from build123d import *

# Parameters (mm, degrees)
F1_DEPTH = 63.5
F0_W     = 25.4
F0_H     = 19.05
F0_H_2   = 9.525
F2_DEPTH = 25.4
F3_DEPTH = 7.9375
F5_R     = 6.35


with BuildPart() as f1:
    # F0 (on Front) → F1 (new body, symmetric)
    with BuildSketch(Plane.XZ):
        Polygon((-41.275, -9.525), (41.275, -9.525), (41.275, 9.525), (22.2237235206, 9.525), (-41.275, 9.525), align=None)
    extrude(amount=F1_DEPTH, both=True)

    # F0 (on Front) → F2 (join, symmetric)
    with BuildSketch(Plane.XZ):
        with BuildLine():
            Line((22.2237235206, 9.525), (41.275, 9.525))
            Line((41.275, 9.525), (40.9650549741, 36.2983668991))
            ThreePointArc((40.9650549741, 36.2983668991), (47.6329246689, 41.7219107909), (56.1502739404, 42.8752))
            Line((56.1502739404, 42.8752), (60.325, 42.8752))
            Line((60.325, 42.8752), (60.325, 61.9252))
            Line((60.325, 61.9252), (50.6626719245, 61.9252))
            ThreePointArc((50.6626719245, 61.9252), (33.3863605767, 55.3894970066), (21.8598589674, 40.95599057))
            Line((21.8598589674, 40.95599057), (22.2237235206, 9.525))
        make_face()
        with Locations((73.025, 52.4002)):
            Rectangle(F0_W, F0_H)
        with Locations((73.025, 38.1127)):
            Rectangle(F0_W, F0_H_2)
    extrude(amount=F2_DEPTH, both=True)

    # F0 (on Front) → F3 (join, symmetric)
    with BuildSketch(Plane.XZ):
        with BuildLine():
            add(Edge.make_bspline(
                [(-41.275, 9.525), (-56.7215932498, 57.9155711565), (13.6268828042, 66.4033379321), (50.6626719245, 61.9252)],
                knots=[0, 0, 0, 0, 105.8220982543, 105.8220982543, 105.8220982543, 105.8220982543], degree=3))
            Line((-41.275, 9.525), (22.2237235206, 9.525))
            Line((22.2237235206, 9.525), (21.8598589674, 40.95599057))
            ThreePointArc((21.8598589674, 40.95599057), (33.3863605767, 55.3894970066), (50.6626719245, 61.9252))
        make_face()
    extrude(amount=F3_DEPTH, both=True)

    # F0 (on Front) → F4 (revolve)
    with BuildSketch(Plane.XZ):
        Polygon((111.125, 61.9252), (85.725, 61.9252), (85.725, 42.8752), (85.725, 33.3502), (111.125, 33.3502), align=None)
    revolve(axis=Axis((85.725, 0, 52.4002), (0, 0, -1)))

    # F5
    f5_edges = [f1.edges().sort_by_distance(p)[0] for p in [
        (41.275, 63.5, 0),
        (-41.275, 63.5, 0),
        (-41.275, -63.5, 0),
        (41.275, -63.5, 0),
    ]]
    fillet(f5_edges, radius=F5_R)


solid = f1.part
Input: part model. Units: mm. Frame: model coordinates. A direction names the side the tool comes from. Round coordinates to 2 decimals unless told otherwise and drop trailing zeros. Order: outer loops, then holes, each group sorted by start corner. A loop starts at its lowest first (then second) coordinate and runs counter-clockwise, first axis right, second up. Notation, with made-up numbers: (29, -10.5) - (77, -10.5) arc R21 cw to (77, 25.5) - close; hole circle Ø6 at (50, 29.5). An arc over 180 degrees is marked (long way). Use a Markdown table: item, result.
1. Section A-A on y = 12. Return the cut outline in (x, z) (3 decimals).
Evaluation:
| item | result |
|---|---|
| outline | (-41.275, -9.525) - (41.275, -9.525) - (41.275, 9.525) - (40.965, 36.298) arc R15.875 cw to (56.15, 42.875) - (60.325, 42.875) - (60.325, 33.35) - (108.112, 33.35) - (108.112, 61.925) - (50.663, 61.925) arc R34.925 ccw to (21.86, 40.956) - (22.224, 9.525) - (-41.275, 9.525) - close |
2. First-contact query: pin 1 (1 mm diameter, centred on x = 52.5, z = 41, fed in from -Y); pin 2 (8 mm diameter, centred on x = 43.5, y = -4, fed in from +Z); pin 3 (1.5 mm diameter, centred on y = 25, z = 32.5, fed in from -X); pin 4 (21 mm diameter, centred on y = 25.5, z = 0, fed in from -X) (3 decimals). Flat tips, straight axial feed; report the tip coordinate or a pass-through.
Evaluation:
| item | result |
|---|---|
| pin 1 | through |
| pin 2 | z = 62.82 |
| pin 3 | x = 21.95 |
| pin 4 | x = -41.275 |
3. Section C-C on x = 63.5. Return the cut outline in (y, z), then the cut area to 3 significant figures.
Evaluation:
| item | result |
|---|---|
| outline | (-25.4, 33.35) - (25.4, 33.35) - (25.4, 61.93) - (-25.4, 61.93) - close |
| area | 1,450 mm^2 |
4. Section D-D on y = -38. Return the cut outline in (x, z) (3 decimals).
Evaluation:
| item | result |
|---|---|
| outline | (-41.275, -9.525) - (41.275, -9.525) - (41.275, 9.525) - (-41.275, 9.525) - close |
5. Section B-B on z = -3.5. Return the cut outline in (x, y) (3 decimals).
Evaluation:
| item | result |
|---|---|
| outline | (-41.275, -57.15) arc R6.35 ccw to (-34.925, -63.5) - (34.925, -63.5) arc R6.35 ccw to (41.275, -57.15) - (41.275, 57.15) arc R6.35 ccw to (34.925, 63.5) - (-34.925, 63.5) arc R6.35 ccw to (-41.275, 57.15) - close |
6. Material intervals for probe 1 along Z at (x, y) = (15, 48) (3 decimals); probe 2 along X at (y, z) = (-53, -1) (3 decimals); probe 3 along Y at (x, z) = (-21, 22), sorted ascending.
Evaluation:
| item | result |
|---|---|
| probe 1 | -9.525 to 9.525 |
| probe 2 | -41.275 to 41.275 |
| probe 3 | -7.94 to 7.94 |
7. Access query for faces 4 (the face through (60.325, 0, 38)), 5 (the face through (33.599, 16.547, 55.543)), 6 (the face through (-2, -7.938, 32)). Directions: +Z, -Z, +X, -X, +Y, -Y. A direction counts if a zero-diameter tool reaches every point of the face in a straight line with its end or side. Return the directions, or none.
Evaluation:
| item | result |
|---|---|
| face 4 | -Z, +Y, -Y |
| face 5 | +Z, -X, +Y |
| face 6 | +Z, -X, -Y |
8. Mould query, pull axis X, two halves, no side actions, for faces 1 (the face through (80, 0, 61.925)), 2 (the face through (41.275, -1, 0)), 3 (the face through (58, 0, 42.875)). Classes: +X half, -X half, draft (parallel to the pull), parting line (faces both ways), or undercut.
Evaluation:
| item | result |
|---|---|
| face 1 | draft |
| face 2 | +X half |
| face 3 | undercut |
